```python
from build123d import *

# Parameters (mm, degrees)
EXTRUDE_1_DEPTH = 2


with BuildPart() as part:
    # 草图2 → 凸台-拉伸1 (new body)
    with BuildSketch(Plane.XY):
        Polygon((-24.246895077, 6.357612039), (-21.746895077, 6.357612039), (-21.746895077, 8.357612039), (-18.146895077, 8.357612039), (-18.146895077, 6.357612039), (71.653104923, 6.357612039), (71.653104923, 8.357612039), (75.253104923, 8.357612039), (75.253104923, 6.357612039), (77.753104923, 6.357612039), (77.753104923, 3.857612039), (76.253104923, 3.857612039), (76.253104923, 1.257612039), (77.753104923, 1.257612039), (77.753104923, -1.742387961), (80.753104923, -1.742387961), (80.753104923, 1.257612039), (82.253104923, 1.257612039), (82.253104923, 3.857612039), (80.753104923, 3.857612039), (80.753104923, 6.357612039), (83.253104923, 6.357612039), (83.253104923, 8.357612039), (86.853104923, 8.357612039), (86.853104923, 6.357612039), (194.993104923, 6.357612039), (194.993104923, 8.357612039), (198.593104923, 8.357612039), (198.593104923, 6.357612039), (201.093104923, 6.357612039), (201.093104923, 3.857612039), (199.593104923, 3.857612039), (199.593104923, 1.257612039), (201.093104923, 1.257612039), (201.093104923, -1.742387961), (204.093104923, -1.742387961), (204.093104923, 1.257612039), (205.593104923, 1.257612039), (205.593104923, 3.857612039), (204.093104923, 3.857612039), (204.093104923, 6.357612039), (206.593104923, 6.357612039), (208.593104923, 6.357612039), (208.593104923, -19.142387961), (206.593104923, -19.142387961), (204.093104923, -19.142387961), (204.093104923, -16.642387961), (205.593104923, -16.642387961), (205.593104923, -14.042387961), (204.093104923, -14.042387961), (204.093104923, -11.042387961), (201.093104923, -11.042387961), (201.093104923, -14.042387961), (199.593104923, -14.042387961), (199.593104923, -16.642387961), (201.093104923, -16.642387961), (201.093104923, -19.142387961), (198.593104923, -19.142387961), (198.593104923, -21.142387961), (194.993104923, -21.142387961), (194.993104923, -19.142387961), (86.853104923, -19.142387961), (86.853104923, -21.142387961), (83.253104923, -21.142387961), (83.253104923, -19.142387961), (80.753104923, -19.142387961), (80.753104923, -16.642387961), (82.253104923, -16.642387961), (82.253104923, -14.042387961), (80.753104923, -14.042387961), (80.753104923, -11.042387961), (77.753104923, -11.042387961), (77.753104923, -14.042387961), (76.253104923, -14.042387961), (76.253104923, -16.642387961), (77.753104923, -16.642387961), (77.753104923, -19.142387961), (75.253104923, -19.142387961), (75.253104923, -21.142387961), (71.653104923, -21.142387961), (71.653104923, -19.142387961), (-18.146895077, -19.142387961), (-18.146895077, -21.142387961), (-21.746895077, -21.142387961), (-21.746895077, -19.142387961), (-24.246895077, -19.142387961), (-24.246895077, -16.642387961), (-22.746895077, -16.642387961), (-22.746895077, -14.042387961), (-24.246895077, -14.042387961), (-24.246895077, -11.042387961), (-27.246895077, -11.042387961), (-27.246895077, -14.042387961), (-28.746895077, -14.042387961), (-28.746895077, -16.642387961), (-27.246895077, -16.642387961), (-27.246895077, -19.142387961), (-29.746895077, -19.142387961), (-29.746895077, -21.142387961), (-33.346895077, -21.142387961), (-33.346895077, 8.357612039), (-29.746895077, 8.357612039), (-29.746895077, 6.357612039), (-27.246895077, 6.357612039), (-27.246895077, 3.857612039), (-28.746895077, 3.857612039), (-28.746895077, 1.257612039), (-27.246895077, 1.257612039), (-27.246895077, -1.742387961), (-24.246895077, -1.742387961), (-24.246895077, 1.257612039), (-22.746895077, 1.257612039), (-22.746895077, 3.857612039), (-24.246895077, 3.857612039), align=None)
        with BuildLine():
            Line((8.47411064, 1.857612039), (68.653104923, 1.857612039))
            ThreePointArc((68.653104923, 1.857612039), (69.360211704, 1.56471882), (69.653104923, 0.857612039))
            Line((69.653104923, 0.857612039), (69.653104923, -12.880354362))
            ThreePointArc((69.653104923, -12.880354362), (69.276579267, -13.662198172), (68.430545438, -13.855273474))
            Line((68.430545438, -13.855273474), (8.251551154, -0.117307073))
            ThreePointArc((8.251551154, -0.117307073), (7.480400644, 0.969596162), (8.47411064, 1.857612039))
        make_face(mode=Mode.SUBTRACT)
        with BuildLine():
            Line((89.853104923, 1.857612039), (163.060529367, 1.857612039))
            ThreePointArc((163.060529367, 1.857612039), (164.056145258, 0.95114811), (163.246781366, -0.124889968))
            Line((163.246781366, -0.124889968), (90.039356922, -14.002753858))
            ThreePointArc((90.039356922, -14.002753858), (89.215238165, -13.79039859), (88.853104923, -13.020251852))
            Line((88.853104923, -13.020251852), (88.853104923, 0.857612039))
            ThreePointArc((88.853104923, 0.857612039), (89.145998142, 1.56471882), (89.853104923, 1.857612039))
        make_face(mode=Mode.SUBTRACT)
        with BuildLine():
            Line((118.785680479, -14.642387961), (191.993104923, -14.642387961))
            ThreePointArc((191.993104923, -14.642387961), (192.700211704, -14.349494742), (192.993104923, -13.642387961))
            Line((192.993104923, -13.642387961), (192.993104923, 0.235475929))
            ThreePointArc((192.993104923, 0.235475929), (192.630971681, 1.005622668), (191.806852924, 1.217977936))
            Line((191.806852924, 1.217977936), (118.599428481, -12.659885955))
            ThreePointArc((118.599428481, -12.659885955), (117.790064588, -13.735924033), (118.785680479, -14.642387961))
        make_face(mode=Mode.SUBTRACT)
        with BuildLine():
            Line((-16.146895077, 0.09557844), (-16.146895077, -13.642387961))
            ThreePointArc((-16.146895077, -13.642387961), (-15.854001858, -14.349494742), (-15.146895077, -14.642387961))
            Line((-15.146895077, -14.642387961), (45.032099206, -14.642387961))
            ThreePointArc((45.032099206, -14.642387961), (46.025809202, -13.754372085), (45.254658692, -12.667468849))
            Line((45.254658692, -12.667468849), (-14.924335591, 1.070497552))
            ThreePointArc((-14.924335591, 1.070497552), (-15.770369421, 0.877422249), (-16.146895077, 0.09557844))
        make_face(mode=Mode.SUBTRACT)
    extrude(amount=EXTRUDE_1_DEPTH)


solid = part.part
```
Could you check a few things on this model? Use its own coordinates, in mm. A direction names the side the tool comes from. Round coordinates to 2 decimals unless told otherwise and drop trailing zeros. Order: outer loops, then holes, each group sorted by start corner. A loop starts at its lowest first (then second) coordinate and runs counter-clockwise, first axis right, second up. Notation, with made-up numbers: M -34.5,-34 L -6.5,-34 A22 cw -6.5,-12 Z; hole C 42.5,87 d4. An arc over 180 degrees is marked long. One line per question, with ' | ' between items. Start each with the question number.
(1) Suppose I cut it at D-D on z = 0.95. Count the separate pieces of the cut face and the enclosed holes in it, then the cut area to 3 significant figures.
(2) For faces 3 (the face through (89, -16, 0)), 4 (the face through (127.156, -6.967, 0.986)), which set-ups out of +Z, -Z, +X, -X, +Y, -Y let a thin tool reach every point of the face, with its end or its side?
(3) For P1, Ø0.6, axis at x = 77, z = 1.5, coming from the +Y side; P2, Ø0.6, axis at y = 7.5, z = 1, coming from the +X side; P3, Ø1, axis at x = 202, z = 1, coming from the +Y side, each with a flat end and sliding along its axis, tell me the tip position at first contact or that it passes through.
(4) Please list where these lines run through material, in increasing order: line 1 along X through (y, z) = (2.5, 0.7); line 2 along X through (y, z) = (7.25, 1.2); line 3 along X through (y, z) = (-18.75, 1.4).
(5) Suppose I cut it at B-B on y = -6.5. List the corners of the cut face in (x, z) for me.
(6) Suppose I cut it at C-C on x = 4.5. List the corners of the cut face in (y, z) for me, then the cut area to 3 significant figures.
(7) Suppose I cut it at A-A on x = 121. List the corners of the cut face in (y, z) for me.
(8) Thinking about a two-plate mould opening in X: for faces 1 (the face through (38.76, -7.08, 0.99)), 2 (the face through (89, -16, 2)), which applies, +X half, -X half, draft (parallel to the pull), parting line (faces both ways), or undercut?
Geometry results:
1) separate pieces: 1 | enclosed holes: 4 | area: 3,600 mm²
2) face 3: -Z, +X, -X, +Y, -Y | face 4: +Z, -Z
3) P1: y = 6.36 | P2: x = 198.59 | P3: y = -1.74
4) line 1: -33.35 to -28.75, -22.75 to 76.25, 82.25 to 199.59, 205.59 to 208.59 | line 2: -33.35 to -29.75, -21.75 to -18.15, 71.65 to 75.25, 83.25 to 86.85, 194.99 to 198.59 | line 3: -33.35 to -27.25, -24.25 to 77.75, 80.75 to 201.09, 204.09 to 208.59
5) outline: M -33.35,0 L -16.15,0 L -16.15,2 L -33.35,2 Z; M 18.24,0 L 36.21,0 L 36.21,2 L 18.24,2 Z; M 69.65,0 L 88.85,0 L 88.85,2 L 69.65,2 Z; M 129.62,0 L 151.09,0 L 151.09,2 L 129.62,2 Z; M 192.99,0 L 208.59,0 L 208.59,2 L 192.99,2 Z
6) outline: M -19.14,0 L -14.64,0 L -14.64,2 L -19.14,2 Z; M -3.36,0 L 6.36,0 L 6.36,2 L -3.36,2 Z | area: 28.4 mm²
7) outline: M -19.14,0 L -14.64,0 L -14.64,2 L -19.14,2 Z; M -12.2,0 L -8.13,0 L -8.13,2 L -12.2,2 Z; M 1.86,0 L 6.36,0 L 6.36,2 L 1.86,2 Z
8) face 1: undercut | face 2: draft
